```python
from build123d import *


with BuildPart() as part:
    # Sketch1 → Revolve1 (revolve)
    with BuildSketch(Plane.XY):
        with BuildLine():
            Line((319.632932386, 0), (319.632932386, 16))
            Line((319.632932386, 16), (313.632932386, 16))
            Line((313.632932386, 16), (313.632932386, 13))
            Line((313.632932386, 13), (-41.367067614, 13))
            Line((-41.367067614, 13), (-41.367067614, 6))
            Line((-41.367067614, 6), (-51.367067614, 6))
            Line((-51.367067614, 6), (-51.367067614, 16))
            ThreePointArc((-51.367067614, 16), (-54.351912619, 8.246211251), (-55.367067614, 0))
            Line((-55.367067614, 0), (319.632932386, 0))
        make_face()
    revolve(axis=Axis((-129.812073534, 0, 0), (1, 0, 0)))


solid = part.part
```
Design review of the part built by this model. Coordinates are the model's own, in mm. Give positions to 0.01 mm unless a question says otherwise; leave off trailing zeros. Loops run counter-clockwise (first coordinate to the right, second up) from the corner with the lowest first, then second, coordinate; pieces in that order, holes last. Notation, with made-up numbers: (72, 18.5) -> (108, 18.5) arc R31 cw to (108, 46.5) -> close; hole circle Ø4 at (29.25, 49.5). An arc over 180 degrees is marked (long way). One line per item, written item: value.
Q1. Draft analysis for pull direction X (two halves, no side actions). For faces 1 (the flat face through (319.633, 0, 0)), 2 (the flat face through (313.633, -1.3, 13.1)), 3 (the cylindrical face through (316.59, -3.47, -15.62)), state which applies: pulls with the +X half, pulls with the -X half, needs draft (parallel to the pull), parting line crosses it, or undercut.
Numbers:
face 1: pulls with the +X half
face 2: undercut
face 3: needs draft
Q2. For L1, parallel to X at y = -7.5, z = 8; L2, parallel to Z at x = 152, y = 1; L3, parallel to X at y = 5.5, z = 3.5, list the stretches that pass through material, from the lowest coordinate up.
Numbers:
L1: x = -53.55 to -51.37, -41.37 to 319.63
L2: z = -12.96 to 12.96
L3: x = -54.74 to -51.37, -41.37 to 319.63
Q3. We need section A-A on y = 0. Give the boundary of the cut face in (x, z).
Numbers:
outline: (-51.37, -16) -> (-51.37, -6) -> (-41.37, -6) -> (-41.37, -13) -> (313.63, -13) -> (313.63, -16) -> (319.63, -16) -> (319.63, 16) -> (313.63, 16) -> (313.63, 13) -> (-41.37, 13) -> (-41.37, 6) -> (-51.37, 6) -> (-51.37, 16) arc R34 ccw to start
Q4. We need section C-C on x = -0.5. Give the boundary of the cut face in (y, z), and give its area (3 significant figures).
Numbers:
outline: circle Ø26 at (0, 0)
area: 531 mm^2
Q5. For pin 1 Ø9.5 at (y, z) = (8, -7.5) entering from -X; pin 2 Ø2 at (x, y) = (163, 4.5) entering from +Z; pin 3 Ø3 at (x, z) = (208, 10.5) entering from -Y; pin 4 Ø10 at (y, z) = (2.5, 0) entering from -X, all flat-tipped, find the tip position at first contact; note any pin that passes through.
Numbers:
pin 1: stops at x = -54.79
pin 2: stops at z = 12.52
pin 3: stops at y = -9.38
pin 4: stops at x = -55.37
